Verification items for the finished model (mm, model axes). Face numbers are marked on the shaded views. A direction names the side the tool comes from. Coordinates: 2 decimals unless noted, no trailing zeros. Order: outer loops, then holes, each group sorted by start corner. A loop starts at its lowest first (then second) coordinate and runs counter-clockwise, first axis right, second up. Notation, with made-up numbers: (-14.5, 65) - (40.5, 65) arc R25 ccw to (40.5, 89) - close; hole circle Ø6 at (49, 41.25). An arc over 180 degrees is marked (long way). Answer as CSV lines item,"result". Start each with the question number.
1. Section check A-A (y = -9.75). Record the cut outline in (x, z), and give its area (3 significant figures).
2. Go/stop test with flat-tipped pins: pin 1 (10 mm diameter, centred on x = 130, z = -36, fed in from -Y); pin 2 (3 mm diameter, centred on y = -4, z = -67, fed in from -X); pin 3 (4 mm diameter, centred on y = -5, z = -10.5, fed in from +X). Record where each tip stops, or that it passes through.
3. Material ranges on L1, parallel to Z at x = 254, y = -0.45; L2, parallel to X at y = -13.25, z = -69.85; L3, parallel to X at y = -3.75, z = -47, recorded low to high. Write a range as [from, to].
4. Section check B-B (z = -39.5). Record the cut outline in (x, y).
5. Section check C-C (x = 172). Record the cut outline in (y, z).
6. Set-up check for the marked faces 1 and 2: record each of +Z, -Z, +X, -X, +Y, -Y from which the full face is reachable in a straight line by a thin tool's end or side.
from build123d import *

# Parameters (mm, degrees)
SKETCH1_W                    = 279.4
SKETCH1_H                    = 76.2
BASE_FLANGE1_DEPTH           = 0.7366
EDGE_FLANGE1_STRIP_W         = 4.4196
EDGE_FLANGE1_STRIP_H         = 0.7366
EDGE_FLANGE1_STRIP_CUT_DEPTH = 76.2
EDGE_FLANGE1_DEPTH           = 76.2
EDGE_FLANGE2_DEPTH           = 76.2
F_6_CLEARANCE_HOLE1_D        = 3.7973
LPATTERN1_COUNT              = 6
LPATTERN1_PITCH              = 45.72
LPATTERN1_COUNT_DIR2         = 2
LPATTERN1_PITCH_DIR2         = 63.5
F_6_CLEARANCE_HOLE2_D        = 3.7973


# Sheet-metal steps are written as plain solids
with BuildPart() as part:
    # Sketch1 → Base-Flange1 (new body)
    with BuildSketch(Plane(origin=(0, 0, 0), x_dir=(1, 0, 0), z_dir=(0, 1, 0))):
        with Locations((139.7, 38.1)):
            Rectangle(SKETCH1_W, SKETCH1_H)
    extrude(amount=-BASE_FLANGE1_DEPTH)

    # Edge-Flange1 strip (across the edge) → Edge-Flange1 strip cut (cut)
    with BuildSketch(Plane(origin=(0, -0.7366, 0), x_dir=(1, 0, 0), z_dir=(0, 0, -1))):
        with Locations((-0.7366, -0.3683)):
            Rectangle(EDGE_FLANGE1_STRIP_W, EDGE_FLANGE1_STRIP_H)
    edge_flange1_strip_cut = extrude(amount=EDGE_FLANGE1_STRIP_CUT_DEPTH, mode=Mode.SUBTRACT)

    # Edge-Flange1 section (across the edge) → Edge-Flange1 (add)
    with BuildSketch(Plane(origin=(0, -0.7366, 0), x_dir=(1, 0, 0), z_dir=(0, 0, -1))):
        with BuildLine():
            Line((0, 0.7366), (0, 11.2268))
            Line((0, 11.2268), (0.7366, 11.2268))
            Line((0.7366, 11.2268), (0.7366, 0.7366))
            ThreePointArc((0.7366, 0.7366), (0.952345145, 0.215745145), (1.4732, 0))
            Line((1.4732, 0), (1.4732, -0.7366))
            ThreePointArc((1.4732, -0.7366), (0.43149029, -0.30510971), (0, 0.7366))
        make_face()
    edge_flange1 = extrude(amount=EDGE_FLANGE1_DEPTH)

    # Edge-Flange2 section (across the edge) → Edge-Flange2 (add)
    with BuildSketch(Plane(origin=(0, -12.7, -76.2), x_dir=(0, 1, 0), z_dir=(0, 0, 1))):
        with BuildLine():
            Line((-0.7366, 0.7366), (-0.7366, 8.1534))
            Line((-0.7366, 8.1534), (0, 8.1534))
            Line((0, 8.1534), (0, 0.7366))
            ThreePointArc((0, 0.7366), (0.215745145, 0.215745145), (0.7366, 0))
            Line((0.7366, 0), (0.7366, -0.7366))
            ThreePointArc((0.7366, -0.7366), (-0.30510971, -0.30510971), (-0.7366, 0.7366))
        make_face()
    edge_flange2 = extrude(amount=EDGE_FLANGE2_DEPTH)

    # Sketch21 → 3/32 (0.09375) Diameter Hole1 (revolve, cut)
    with BuildSketch(Plane(origin=(25.4, 0, -69.85), x_dir=(0, 0, 1), z_dir=(1, 0, 0))):
        Polygon((0, 0), (0, 2.167399349), (2.38125, 0.7366), (2.38125, 0), align=None)
    f_3_32_0_09375_diameter_hole1 = revolve(axis=Axis((25.4, 6.35, -69.85), (0, -1, 0)), mode=Mode.SUBTRACT)

    # #6 Clearance Hole1 (through all)
    with Locations(Plane(origin=(0, -12.7, 0), x_dir=(1, 0, 0), z_dir=(0, 1, 0))):
        with Locations((-4.445, 69.85), (-4.445, 6.35)):
            f_6_clearance_hole1 = Hole(F_6_CLEARANCE_HOLE1_D / 2)

    # LPattern1: 3_32 _0.09375_ Diameter Hole1 6 × 2
    with Locations(*[(i * LPATTERN1_PITCH, 0, j * LPATTERN1_PITCH_DIR2) for i in range(LPATTERN1_COUNT) for j in range(LPATTERN1_COUNT_DIR2) if (i, j) != (0, 0)]):
        add(f_3_32_0_09375_diameter_hole1, mode=Mode.SUBTRACT)

    # Mirror2: Edge-Flange1 strip cut, Edge-Flange1, Edge-Flange2, #6 Clearance Hole1 across plane
    add(edge_flange1_strip_cut.mirror(Plane.ZY.offset(-139.7)), mode=Mode.SUBTRACT)
    add(edge_flange1.mirror(Plane.ZY.offset(-139.7)))
    add(edge_flange2.mirror(Plane.ZY.offset(-139.7)))
    add(f_6_clearance_hole1.mirror(Plane.ZY.offset(-139.7)), mode=Mode.SUBTRACT)

    # #6 Clearance Hole2 (through all)
    with Locations(Plane(origin=(0, 0, 0), x_dir=(1, 0, 0), z_dir=(0, 1, 0))):
        with Locations((139.7, 69.85), (139.7, 6.35)):
            Hole(F_6_CLEARANCE_HOLE2_D / 2)


solid = part.part
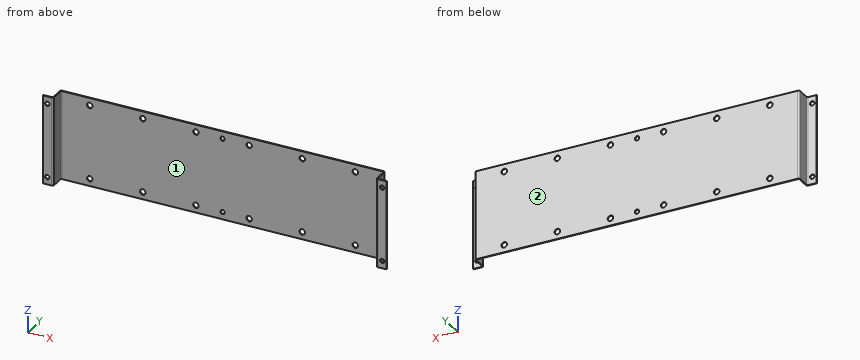
Evaluation:
1,outline,"(0, -76.2) - (0.74, -76.2) - (0.74, 0) - (0, 0) - close; (278.66, -76.2) - (279.4, -76.2) - (279.4, 0) - (278.66, 0) - close"
1,area,"112 mm²"
2,pin 1,"stops at y = -0.74"
2,pin 2,"stops at x = 0"
2,pin 3,"stops at x = 279.4"
3,L1,"z = [-76.2, -72.23], [-67.47, -8.73], [-3.97, 0]"
3,L2,"x = [-8.15, -6.34], [-2.55, -0.02], [279.42, 281.95], [285.74, 287.55]"
3,L3,"x = [0, 0.74], [278.66, 279.4]"
4,outline,"(-8.15, -13.44) - (-0.74, -13.44) arc R1.47 ccw to (0.74, -11.96) - (0.74, -1.47) arc R0.74 cw to (1.47, -0.74) - (277.93, -0.74) arc R0.74 cw to (278.66, -1.47) - (278.66, -11.96) arc R1.47 ccw to (280.14, -13.44) - (287.55, -13.44) - (287.55, -12.7) - (280.14, -12.7) arc R0.74 cw to (279.4, -11.96) - (279.4, -1.47) arc R1.47 ccw to (277.93, 0) - (1.47, 0) arc R1.47 ccw to (0, -1.47) - (0, -11.96) arc R0.74 cw to (-0.74, -12.7) - (-8.15, -12.7) - close"
5,outline,"(-0.74, -76.2) - (0, -76.2) - (0, 0) - (-0.74, 0) - close"
6,face 1,"+Z, -Z, -Y"
6,face 2,"+Z, -Z, +X, -X, +Y"
